For this review, take the finished solid that the model builds, in its own axes (mm). A direction names the side the tool comes from. Coordinates: 2 decimals unless noted, no trailing zeros. Order: outer loops, then holes, each group sorted by start corner. A loop starts at its lowest first (then second) coordinate and runs counter-clockwise, first axis right, second up. Notation, with made-up numbers: (71.5, 82.25) -> (82.5, 82.25) arc R12 ccw to (82.5, 101.25) -> close; hole circle Ø3 at (-18, -29). An arc over 180 degrees is marked (long way). Write item = value, one per line. Start each with the question number.
1) Machinability: for faces 1 (the face through (47.8, 5.25, 42.7)), 2 (the face through (-103, 5.25, -68)), 3 (the face through (44.326, 51, -67)), 4 (the face through (-97.274, 51, 46)), which of the approach directions +Z, -Z, +X, -X, +Y, -Y give a long, thin tool a straight path to every point of the face, cutting with its end or side? Answer none if there is none.
2) Wall thickness on probe 1 along X at (y, z) = (20, 21); probe 2 along X at (y, z) = (53, -64.5): over which ranges is each line inside the solid? List them lowest first. Write a range as [from, to].
3) Consider section A-A on y = 86.5. Give the boundary of the cut face in (x, z), and give its area (3 significant figures).
4) Draft analysis for pull direction X (two halves, no side actions). For faces 5 (the face through (-103, 51, 40.222)), 6 (the face through (46.876, 2.662, -66.433)), 7 (the face through (-97.274, 51, -67)), state which applies: +X half, -X half, draft (parallel to the pull), parting line (faces both ways), or undercut.
5) Insertion check: pin 1 Ø5.5 at (x, z) = (-101.87, -65.98) entering from +Y; pin 2 Ø2 at (y, z) = (36, -68.5) entering from -X; pin 3 Ø3.5 at (y, z) = (32, 46.5) entering from +X; pin 4 Ø3 at (x, z) = (-25, 28) entering from -Y. Each pin has a flat end and moves straight along its axis. Give the tip position at first contact, or say it passes through.
6) Consider section B-B on y = 51. Give the boundary of the cut face in (x, z), and give its area (3 significant figures).
from build123d import *

# Parameters (mm, degrees)
DODANIE_WYCI_GNI_CIE1_DEPTH = 95
WYTNIJ_WYCI_GNI_CIE2_DEPTH  = 89.75
SZKIC6_R                    = 2.1
WYTNIJ_WYCI_GNI_CIE4_DEPTH  = 5.25
SZKIC7_W                    = 90
SZKIC7_H                    = 55.75
WYTNIJ_WYCI_GNI_CIE6_DEPTH  = 1


with BuildPart() as part:
    # Szkic1 → Dodanie-wyciągnięcie1 (new body)
    with BuildSketch(Plane(origin=(0, 0, 0), x_dir=(1, 0, 0), z_dir=(0, 1, 0))):
        with BuildLine():
            Line((-103.973988439, 70.578034682), (51.026011561, 70.578034682))
            ThreePointArc((51.026011561, 70.578034682), (52.793778514, 69.845801635), (53.526011561, 68.078034682))
            Line((53.526011561, 68.078034682), (53.526011561, -46.921965318))
            ThreePointArc((53.526011561, -46.921965318), (52.793778514, -48.689732271), (51.026011561, -49.421965318))
            Line((51.026011561, -49.421965318), (-103.973988439, -49.421965318))
            ThreePointArc((-103.973988439, -49.421965318), (-105.741755392, -48.689732271), (-106.473988439, -46.921965318))
            Line((-106.473988439, -46.921965318), (-106.473988439, 68.078034682))
            ThreePointArc((-106.473988439, 68.078034682), (-105.741755392, 69.845801635), (-103.973988439, 70.578034682))
        make_face()
    extrude(amount=DODANIE_WYCI_GNI_CIE1_DEPTH)

    # Szkic3 → Wytnij-wyciągnięcie2 (cut)
    with BuildSketch(Plane(origin=(0, 95, 0), x_dir=(1, 0, 0), z_dir=(0, 1, 0))):
        with BuildLine():
            Line((53.526011561, 70.578034682), (53.526011561, 61.378034682))
            Line((53.526011561, 61.378034682), (46.826011561, 61.378034682))
            ThreePointArc((46.826011561, 61.378034682), (45.058244608, 62.110267729), (44.326011561, 63.878034682))
            Line((44.326011561, 63.878034682), (44.326011561, 70.578034682))
            Line((44.326011561, 70.578034682), (53.526011561, 70.578034682))
        make_face()
        with BuildLine():
            Line((-97.273988439, 63.878034682), (-97.273988439, 70.578034682))
            Line((-97.273988439, 70.578034682), (-106.473988439, 70.578034682))
            Line((-106.473988439, 70.578034682), (-106.473988439, 61.378034682))
            Line((-106.473988439, 61.378034682), (-99.773988439, 61.378034682))
            ThreePointArc((-99.773988439, 61.378034682), (-98.006221486, 62.110267729), (-97.273988439, 63.878034682))
        make_face()
        with BuildLine():
            Line((-106.473988439, -49.421965318), (-106.473988439, -40.221965318))
            Line((-106.473988439, -40.221965318), (-99.773988439, -40.221965318))
            ThreePointArc((-99.773988439, -40.221965318), (-98.006221486, -40.954198365), (-97.273988439, -42.721965318))
            Line((-97.273988439, -42.721965318), (-97.273988439, -49.421965318))
            Line((-97.273988439, -49.421965318), (-106.473988439, -49.421965318))
        make_face()
        with BuildLine():
            Line((44.326011561, -42.721965318), (44.326011561, -49.421965318))
            Line((44.326011561, -49.421965318), (53.526011561, -49.421965318))
            Line((53.526011561, -49.421965318), (53.526011561, -40.221965318))
            Line((53.526011561, -40.221965318), (46.826011561, -40.221965318))
            ThreePointArc((46.826011561, -40.221965318), (45.058244608, -40.954198365), (44.326011561, -42.721965318))
        make_face()
    extrude(amount=-WYTNIJ_WYCI_GNI_CIE2_DEPTH, mode=Mode.SUBTRACT)

    # Szkic6 → Wytnij-wyciągnięcie4 (cut)
    with BuildSketch(Plane(origin=(0, 5.25, 0), x_dir=(1, 0, 0), z_dir=(0, 1, 0))):
        with Locations(Location((48.926011561, 65.978034682, 0), (0, 0, 270))):
            Circle(SZKIC6_R)
        with Locations(Location((-101.873988439, 65.978034682, 0), (0, 0, 270))):
            Circle(SZKIC6_R)
        with Locations(Location((-101.873988439, -44.821965318, 0), (0, 0, 270))):
            Circle(SZKIC6_R)
        with Locations(Location((48.926011561, -44.821965318, 0), (0, 0, 270))):
            Circle(SZKIC6_R)
    extrude(amount=-WYTNIJ_WYCI_GNI_CIE4_DEPTH, mode=Mode.SUBTRACT)

    # Szkic7 → Wytnij-wyciągnięcie6 (cut)
    with BuildSketch(Plane.ZY.offset(106.473988439)):
        with Locations((-10.578034682, 33.125)):
            Rectangle(SZKIC7_W, SZKIC7_H)
    extrude(amount=-WYTNIJ_WYCI_GNI_CIE6_DEPTH, mode=Mode.SUBTRACT)


solid = part.part
Answer sheet:
q1.face_1 = +Z, +X, +Y
q1.face_2 = -Z, -X, +Y
q1.face_3 = -Z, +X, +Y
q1.face_4 = +Z, -X, +Y
q2.probe_1 = [-105.47, 53.53]
q2.probe_2 = [-97.27, 44.33]
q3.outline = (-106.47, -61.38) -> (-99.77, -61.38) arc R2.5 cw to (-97.27, -63.88) -> (-97.27, -70.58) -> (44.33, -70.58) -> (44.33, -63.88) arc R2.5 cw to (46.83, -61.38) -> (53.53, -61.38) -> (53.53, 40.22) -> (46.83, 40.22) arc R2.5 cw to (44.33, 42.72) -> (44.33, 49.42) -> (-97.27, 49.42) -> (-97.27, 42.72) arc R2.5 cw to (-99.77, 40.22) -> (-106.47, 40.22) -> close
q3.area = 18,900 mm2
q4.face_5 = draft
q4.face_6 = undercut
q4.face_7 = -X half
q5.pin_1 = 5.25
q5.pin_2 = -97.27
q5.pin_3 = 44.33
q5.pin_4 = 0
q6.outline = (-106.47, -61.38) -> (-99.77, -61.38) arc R2.5 cw to (-97.27, -63.88) -> (-97.27, -70.58) -> (44.33, -70.58) -> (44.33, -63.88) arc R2.5 cw to (46.83, -61.38) -> (53.53, -61.38) -> (53.53, 40.22) -> (46.83, 40.22) arc R2.5 cw to (44.33, 42.72) -> (44.33, 49.42) -> (-97.27, 49.42) -> (-97.27, 42.72) arc R2.5 cw to (-99.77, 40.22) -> (-106.47, 40.22) -> (-106.47, 34.42) -> (-105.47, 34.42) -> (-105.47, -55.58) -> (-106.47, -55.58) -> close
q6.area = 18,800 mm2
